from build123d import *

# Parameters (mm, degrees)
SKETCH2_W               = 80
SKETCH2_H               = 47.65
BOSS_EXTRUDE1_DEPTH     = 3.175
SKETCH3_W               = 15
SKETCH3_H               = 3.5
BOSS_EXTRUDE2_DEPTH     = 3.175
SKETCH4_W               = 3.5
SKETCH4_H               = 26.9
BOSS_EXTRUDE3_DEPTH     = 3.175
SKETCH5_R               = 1.5
CUT_EXTRUDE1_DEPTH      = 20
LPATTERN1_COUNT         = 3
LPATTERN1_PITCH         = 12.8
MIRROR3_COPY_1_SKETCH_R = 1.5
MIRROR3_COPY_1_DEPTH    = 20
MIRROR3_COPY_2_SKETCH_R = 1.5
MIRROR3_COPY_2_DEPTH    = 20
SKETCH6_W               = 15
SKETCH6_H               = 30
CUT_EXTRUDE2_DEPTH      = 52.468303353
FILLET1_R               = 2.5
CUT_EXTRUDE3_DEPTH      = 52.468303353
CUT_EXTRUDE3_DEPTH_BACK = 52.468303353
SKETCH7_R               = 2.05


with BuildPart() as part:
    # Sketch2 → Boss-Extrude1 (new body)
    with BuildSketch(Plane(origin=(0, 0, 0), x_dir=(1, 0, 0), z_dir=(0, 1, 0))):
        Rectangle(SKETCH2_W, SKETCH2_H)
    extrude(amount=BOSS_EXTRUDE1_DEPTH)

    # Sketch3 → Boss-Extrude2 (add)
    with BuildSketch(Plane(origin=(0, 3.175, 0), x_dir=(1, 0, 0), z_dir=(0, 1, 0))):
        with Locations((0, 25.575)):
            Rectangle(SKETCH3_W, SKETCH3_H)
    boss_extrude2 = extrude(amount=-BOSS_EXTRUDE2_DEPTH)

    # Sketch4 → Boss-Extrude3 (add)
    with BuildSketch(Plane(origin=(0, 3.175, 0), x_dir=(1, 0, 0), z_dir=(0, 1, 0))):
        with Locations((-41.75, 0)):
            Rectangle(SKETCH4_W, SKETCH4_H)
    boss_extrude3 = extrude(amount=-BOSS_EXTRUDE3_DEPTH)

    # Mirror1: Boss-Extrude3 across plane
    add(boss_extrude3.mirror(Plane(origin=(0, 0, 0), x_dir=(0, 0, 1), z_dir=(1, 0, 0))))

    # Mirror2: Boss-Extrude2 across plane
    add(boss_extrude2.mirror(Plane.XY))

    # Sketch5 → Cut-Extrude1 (cut)
    with BuildSketch(Plane(origin=(0, 3.175, 0), x_dir=(1, 0, 0), z_dir=(0, 1, 0))):
        with Locations(Location((-30.2, 7.95, 0), (0, 0, 270))):
            Circle(SKETCH5_R)
    cut_extrude1 = extrude(amount=-CUT_EXTRUDE1_DEPTH, mode=Mode.SUBTRACT)

    # LPattern1: Cut-Extrude1 ×3
    with Locations(*[(i * LPATTERN1_PITCH, 0, 0) for i in range(1, LPATTERN1_COUNT)]):
        add(cut_extrude1, mode=Mode.SUBTRACT)

    # Mirror3: Cut-Extrude1 across plane
    add(cut_extrude1.mirror(Plane.XY), mode=Mode.SUBTRACT)

    # Mirror3 copy 1 sketch → Mirror3 copy 1 (cut)
    with BuildSketch(Plane(origin=(12.8, 3.175, 0), x_dir=(1, 0, 0), z_dir=(0, 1, 0))):
        with Locations((-30.2, -7.95)):
            Circle(MIRROR3_COPY_1_SKETCH_R)
    extrude(amount=-MIRROR3_COPY_1_DEPTH, mode=Mode.SUBTRACT)

    # Mirror3 copy 2 sketch → Mirror3 copy 2 (cut)
    with BuildSketch(Plane(origin=(25.6, 3.175, 0), x_dir=(1, 0, 0), z_dir=(0, 1, 0))):
        with Locations((-30.2, -7.95)):
            Circle(MIRROR3_COPY_2_SKETCH_R)
    extrude(amount=-MIRROR3_COPY_2_DEPTH, mode=Mode.SUBTRACT)

    # Sketch6 → Cut-Extrude2 (cut, through all)
    with BuildSketch(Plane(origin=(0, 3.175, 0), x_dir=(1, 0, 0), z_dir=(0, 1, 0))):
        with Locations((23.5, 0)):
            Rectangle(SKETCH6_W, SKETCH6_H)
    extrude(amount=-CUT_EXTRUDE2_DEPTH, mode=Mode.SUBTRACT)

    # Fillet1
    fillet1_edges = [part.edges().sort_by_distance(p)[0] for p in [
        (16, 1.5875, 15),
        (16, 1.5875, -15),
        (31, 1.5875, -15),
        (31, 1.5875, 15),
    ]]
    fillet(fillet1_edges, radius=FILLET1_R)

    # Sketch7 → Cut-Extrude3 (cut, two sides: drawn at the far end of the back side and taken through both)
    with BuildSketch(Plane(origin=(0, 3.175, 0), x_dir=(1, 0, 0), z_dir=(0, 1, 0)).offset(-CUT_EXTRUDE3_DEPTH_BACK)):
        with Locations(Location((-35, 18.825, 0), (0, 0, 270))):
            Circle(SKETCH7_R)
        with Locations(Location((35, 18.825, 0), (0, 0, 270))):
            Circle(SKETCH7_R)
        with Locations(Location((-35, -18.825, 0), (0, 0, 270))):
            Circle(SKETCH7_R)
        with Locations(Location((35, -18.825, 0), (0, 0, 270))):
            Circle(SKETCH7_R)
    extrude(amount=CUT_EXTRUDE3_DEPTH + CUT_EXTRUDE3_DEPTH_BACK, mode=Mode.SUBTRACT)


solid = part.part
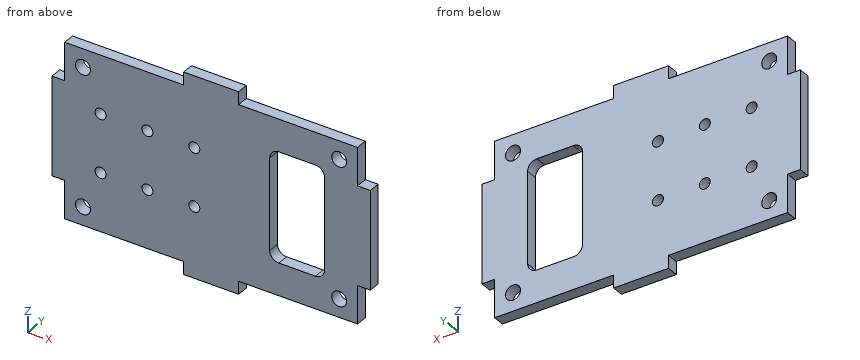
Design review of the part built by this model. Coordinates are the model's own, in mm. Give positions to 0.01 mm unless a question says otherwise; leave off trailing zeros. Order: outer loops, then holes, each group sorted by start corner. A loop starts at its lowest first (then second) coordinate and runs counter-clockwise, first axis right, second up.
1. Add section D-D, the plane z = -19. State the section outline as (x, y) points (3 decimals).
Solution:
outline: (-40, 0) - (-37.043, 0) - (-37.043, 3.175) - (-40, 3.175) - close; (-32.957, 0) - (32.957, 0) - (32.957, 3.175) - (-32.957, 3.175) - close; (37.043, 0) - (40, 0) - (40, 3.175) - (37.043, 3.175) - close
2. For pin 1 Ø1 at (x, y) = (-41.5, 1.5) entering from -Z; pin 2 Ø1.6 at (y, z) = (1.5, -16) entering from +X; pin 3 Ø1.8 at (x, z) = (-30.2, -7.95) entering from -Y; pin 4 Ø1 at (y, z) = (1, -24.5) entering from +X, all flat-tipped, find the tip position at first contact; note any pin that passes through.
Solution:
pin 1: stops at z = -13.45
pin 2: stops at x = 40
pin 3: passes through
pin 4: stops at x = 7.5
3. Add section B-B, the plane x = 35. State the section outline as (y, z) points (3 decimals), then the cut area to 3 significant figures.
Solution:
outline: (0, -23.825) - (3.175, -23.825) - (3.175, -20.875) - (0, -20.875) - close; (0, -16.775) - (3.175, -16.775) - (3.175, 16.775) - (0, 16.775) - close; (0, 20.875) - (3.175, 20.875) - (3.175, 23.825) - (0, 23.825) - close
area: 125 mm2
4. Add section A-A, the plane z = -7.95. State the section outline as (x, y) points (3 decimals), then the cut area to 3 significant figures.
Solution:
outline: (-43.5, 0) - (-31.7, 0) - (-31.7, 3.175) - (-43.5, 3.175) - close; (-28.7, 0) - (-18.9, 0) - (-18.9, 3.175) - (-28.7, 3.175) - close; (-15.9, 0) - (-6.1, 0) - (-6.1, 3.175) - (-15.9, 3.175) - close; (-3.1, 0) - (16, 0) - (16, 3.175) - (-3.1, 3.175) - close; (31, 0) - (43.5, 0) - (43.5, 3.175) - (31, 3.175) - close
area: 200 mm2
5. To check wall thickness, follow L1, parallel to X at y = 1.3, z = 7.95; L2, parallel to Z at x = -35, y = 0.8 (3 decimals); L3, parallel to Z at x = 26, y = 3 (3 decimals). State the ranges of each line that lie inside material, in increasing order.
Solution:
L1: x = -43.5 to -31.7, -28.7 to -18.9, -15.9 to -6.1, -3.1 to 16, 31 to 43.5
L2: z = -23.825 to -20.875, -16.775 to 16.775, 20.875 to 23.825
L3: z = -23.825 to -15, 15 to 23.825
6. Add section C-C, the plane x = 25.5. State the section outline as (y, z) points (3 decimals), then the cut area to 3 significant figures.
Solution:
outline: (0, -23.825) - (3.175, -23.825) - (3.175, -15) - (0, -15) - close; (0, 15) - (3.175, 15) - (3.175, 23.825) - (0, 23.825) - close
area: 56.0 mm2
